from build123d import *

# Parameters (mm, degrees)
SKETCH1_W           = 80
SKETCH1_H           = 80
BOSS_EXTRUDE1_DEPTH = 2
SKETCH2_R           = 3.5
BOSS_EXTRUDE2_DEPTH = 1
SKETCH3_R           = 2
CUT_EXTRUDE1_DEPTH  = 1
FILLET1_R           = 5
SKETCH4_R           = 2
CUT_EXTRUDE2_DEPTH  = 11
SKETCH5_W           = 60
SKETCH5_H           = 60
CUT_EXTRUDE4_DEPTH  = 1


with BuildPart() as part:
    # Sketch1 → Boss-Extrude1 (new body)
    with BuildSketch(Plane.XY):
        Rectangle(SKETCH1_W, SKETCH1_H)
    extrude(amount=BOSS_EXTRUDE1_DEPTH)

    # Sketch2 → Boss-Extrude2 (add)
    with BuildSketch(Plane(origin=(0, 0, 0), x_dir=(-1, 0, 0), z_dir=(0, 0, -1))):
        with Locations(Location((0, 24.55, 0), (0, 0, 116.872206362))):
            Circle(SKETCH2_R)
        with Locations(Location((24.55, 0, 0), (0, 0, 26.872206362))):
            Circle(SKETCH2_R)
        with Locations(Location((0, -24.55, 0), (0, 0, 243.127793638))):
            Circle(SKETCH2_R)
        with Locations(Location((-24.55, 0, 0), (0, 0, 153.127793638))):
            Circle(SKETCH2_R)
    extrude(amount=BOSS_EXTRUDE2_DEPTH)

    # Sketch3 → Cut-Extrude1 (cut)
    with BuildSketch(Plane(origin=(0, 0, -1), x_dir=(-1, 0, 0), z_dir=(0, 0, -1))):
        with Locations((-24.55, 0)):
            Circle(SKETCH3_R)
        with Locations((0, 24.55)):
            Circle(SKETCH3_R)
        with Locations((0, -24.55)):
            Circle(SKETCH3_R)
        with Locations((24.55, 0)):
            Circle(SKETCH3_R)
    extrude(amount=-CUT_EXTRUDE1_DEPTH, mode=Mode.SUBTRACT)

    # Fillet1
    fillet1_edges = [part.edges().sort_by_distance(p)[0] for p in [
        (-40, 40, 1),
        (40, 40, 1),
        (-40, -40, 1),
        (40, -40, 1),
    ]]
    fillet(fillet1_edges, radius=FILLET1_R)

    # Sketch4 → Cut-Extrude2 (cut)
    with BuildSketch(Plane.XY.offset(2)):
        with Locations((35, 35)):
            Circle(SKETCH4_R)
        with Locations((-35, 35)):
            Circle(SKETCH4_R)
        with Locations((35, -35)):
            Circle(SKETCH4_R)
        with Locations((-35, -35)):
            Circle(SKETCH4_R)
    extrude(amount=-CUT_EXTRUDE2_DEPTH, mode=Mode.SUBTRACT)

    # Sketch5 → Cut-Extrude4 (cut)
    with BuildSketch(Plane(origin=(0, 0, 0), x_dir=(-1, 0, 0), z_dir=(0, 0, -1))):
        Rectangle(SKETCH5_W, SKETCH5_H)
        with BuildLine():
            Line((26.464466094, -3.535533906), (3.535533906, -26.464466094))
            ThreePointArc((3.535533906, -26.464466094), (0, -27.928932188), (-3.535533906, -26.464466094))
            Line((-3.535533906, -26.464466094), (-26.464466094, -3.535533906))
            ThreePointArc((-26.464466094, -3.535533906), (-27.928932188, 0), (-26.464466094, 3.535533906))
            Line((-26.464466094, 3.535533906), (-3.535533906, 26.464466094))
            ThreePointArc((-3.535533906, 26.464466094), (0, 27.928932188), (3.535533906, 26.464466094))
            Line((3.535533906, 26.464466094), (26.464466094, 3.535533906))
            ThreePointArc((26.464466094, 3.535533906), (27.928932188, 0), (26.464466094, -3.535533906))
        make_face(mode=Mode.SUBTRACT)
    extrude(amount=-CUT_EXTRUDE4_DEPTH, mode=Mode.SUBTRACT)


solid = part.part
Here's how the part is built. I have some questions about the finished solid (model axes, mm). A direction names the side the tool comes from. Coordinates: 2 decimals unless noted, no trailing zeros. Order: outer loops, then holes, each group sorted by start corner. A loop starts at its lowest first (then second) coordinate and runs counter-clockwise, first axis right, second up. Notation, with made-up numbers: (-38, 14.25) - (-19, 14.25) arc R19 ccw to (-19, 24.25) - close; hole circle Ø10 at (-0.5, 52). An arc over 180 degrees is marked (long way). Use CSV: the item, a comma, the result in double quotes. Start each with the question number.
1. If we mould it in two halves opening along Y, with no side actions, what happens to faces 3 (the face through (38, 39, 1)), 4 (the face through (25, 0, 0)), 5 (the face through (-27, -1, -1)), 6 (the face through (15.2, 14.8, 0.5))? For each: +Y half, -Y half, draft (parallel to the pull), parting line (faces both ways), or undercut.
2. I'm going to push flat-ended pins straight in: pin 1 (4.5 mm diameter, centred on x = 1, y = 25, fed in from -Z); pin 2 (16.5 mm diameter, centred on x = 12.5, y = 0.5, fed in from -Z); pin 3 (3 mm diameter, centred on x = 35, y = 35, fed in from -Z); pin 4 (1.5 mm diameter, centred on x = -11.5, y = -25.5, fed in from -Z). Where does each tip first touch, or does it pass through?
3. Suppose I cut it at A-A on y = -19. List the corners of the cut face in (x, z) for me, then the cut area to 3 significant figures.
4. Please list where these lines run through material, in increasing order: line 1 (Y direction, x = 0, z = -0.15); line 2 (Y direction, x = 24.55, z = -0.7); line 3 (Y direction, x = 35, z = 1.4). Write a range as from..to.
5. For faces 1 (the face through (1, -27, -1)), 2 (the face through (-22.552, 0.088, -0.507)), which set-ups out of +Z, -Z, +X, -X, +Y, -Y let a thin tool reach every point of the face, with its end or its side?
6. Suppose I cut it at C-C on y = 24.55. List the corners of the cut face in (x, z) for me.
7. Suppose I cut it at B-B on x = 0. List the corners of the cut face in (y, z) for me, then the cut area to 3 significant figures.
Output:
1,face 3,"+Y half"
1,face 4,"undercut"
1,face 5,"draft"
1,face 6,"undercut"
2,pin 1,"stops at z = -1"
2,pin 2,"stops at z = 0"
2,pin 3,"passes through"
2,pin 4,"stops at z = 1"
3,outline,"(-40, 0) - (-30, 0) - (-30, 1) - (-11, 1) - (-11, 0) - (11, 0) - (11, 1) - (30, 1) - (30, 0) - (40, 0) - (40, 2) - (-40, 2) - close"
3,area,"122 mm2"
4,line 1,"y = -28.05..-26.55, -22.55..-21.05, 21.05..22.55, 26.55..28.05"
4,line 2,"y = -3.5..-2, 2..3.5"
4,line 3,"y = -40..-37, -33..33, 37..40"
5,face 1,"-Z, +X, -X, +Y, -Y"
5,face 2,"-Z"
6,outline,"(-40, 0) - (-30, 0) - (-30, 1) - (-5.45, 1) - (-5.45, 0) - (-3.5, 0) - (-3.5, -1) - (-2, -1) - (-2, 0) - (2, 0) - (2, -1) - (3.5, -1) - (3.5, 0) - (5.45, 0) - (5.45, 1) - (30, 1) - (30, 0) - (40, 0) - (40, 2) - (-40, 2) - close"
7,outline,"(-40, 0) - (-30, 0) - (-30, 1) - (-27.93, 1) - (-27.93, 0) - (-28.05, 0) - (-28.05, -1) - (-26.55, -1) - (-26.55, 0) - (-22.55, 0) - (-22.55, -1) - (-21.05, -1) - (-21.05, 0) - (21.05, 0) - (21.05, -1) - (22.55, -1) - (22.55, 0) - (26.55, 0) - (26.55, -1) - (28.05, -1) - (28.05, 0) - (27.93, 0) - (27.93, 1) - (30, 1) - (30, 0) - (40, 0) - (40, 2) - (-40, 2) - close"
7,area,"162 mm2"
